Autodesk Inventor part; units mm, degrees
ref_plane "YZ Plane" through (0, 0, 0) normal (1, 0, 0) x (0, 1, 0)
ref_plane "XZ Plane" through (0, 0, 0) normal (0, 1, 0) x (-1, 0, 0)
ref_plane "XY Plane" through (0, 0, 0) normal (0, 0, 1) x (1, 0, 0)
sketch "main" plane through (0, 0, 0) normal (0, 0, 1) x (1, 0, 0)
  circle A0 centre (-11.9584, 56.4908) radius 2.1844
  circle A1 centre (13.4416, 56.4908) radius 2.1844
  circle A2 centre (13.4416, -57.8092) radius 2.1844
  circle A3 centre (-11.9584, -57.8092) radius 2.1844
  arc A4 (19.7916, 56.4908) -> (13.4416, 62.8408) centre (13.4416, 56.4908) ccw
  arc A5 (-11.9584, 62.8408) -> (-18.3084, 56.4908) centre (-11.9584, 56.4908) ccw
  arc A6 (-18.3084, -57.8092) -> (-11.9584, -64.1592) centre (-11.9584, -57.8092) ccw
  arc A7 (13.4416, -64.1592) -> (19.7916, -57.8092) centre (13.4416, -57.8092) ccw
  line L0 (13.4416, 62.8408) -> (-11.9584, 62.8408)
  line L1 (-18.3084, 56.4908) -> (-18.3084, -57.8092)
  line L2 (-11.9584, -64.1592) -> (13.4416, -64.1592)
  line L3 (19.7916, -57.8092) -> (19.7916, 56.4908)
  point P0 (0.7416, -0.6592)
  dimension "d0" = 12.7
  dimension "d1" = 12.7
  dimension "d2" = 12.7
  dimension "d3" = 12.7
sketch "Sketch1" plane through (0, 0, 0) normal (0, 1, 0) x (-1, 0, 0)
  circle A0 centre (-25.4, 0) radius 2.1844
  circle A1 centre (0, 0) radius 2.1844
  circle A2 centre (0, -114.3) radius 2.1844
  circle A3 centre (-25.4, -114.3) radius 2.1844
  arc A4 (6.35, 0) -> (0, 6.35) centre (0, 0) ccw
  arc A5 (-25.4, 6.35) -> (-31.75, 0) centre (-25.4, 0) ccw
  arc A6 (-31.75, -114.3) -> (-25.4, -120.65) centre (-25.4, -114.3) ccw
  arc A7 (0, -120.65) -> (6.35, -114.3) centre (0, -114.3) ccw
  line L0 (0, 6.35) -> (-25.4, 6.35)
  line L1 (-31.75, 0) -> (-31.75, -114.3)
  line L2 (-25.4, -120.65) -> (0, -120.65)
  line L3 (6.35, -114.3) -> (6.35, 0)
extrude "Extrusion1" add sketch "Sketch1" along normal blind 1.5875
properties part number "Brace Gusset" material "Acetal Resin, White"
Part model, mm, in its own coordinate system. Round coordinates to 2 decimals unless told otherwise and drop trailing zeros. Write each loop counter-clockwise with the first axis right and the second up, starting at its lowest first coordinate (ties: lowest second). Pieces come first, ordered by that corner, then holes. Notation, with made-up numbers: M -12.75,62 L -1.75,62 A26 cw -1.75,91 Z; hole C -27.75,56.25 d2. An arc over 180 degrees is marked long. Return JSON: item names as keys, results as strings. Group by question number.
(1) Two-plate mould, pull along X, no slides. Class faces 1 (the face through (13, 1.588, -56)), 2 (the face through (-4.44, 0.78, 4.54)), 3 (the face through (23.382, 0.783, 0.837)): +X half, -X half, draft (parallel to the pull), parting line (faces both ways), or undercut.
(2) Drill centre line: probe 1 along Z at (x, y) = (0, 0.6). Where is it in solid material? Low to high.
(3) Saw through at A-A on y = 0.8. Write the cut outline in (x, z).
(4) Pin check, flat tip, straight feed: pin 1 Ø7 at (x, z) = (25.4, -114.3) entering from +Y. Stop position of the tip, or through.
Returned:
{
 "1": {"face 1": "draft", "face 2": "-X half", "face 3": "undercut"},
 "2": {"probe 1": "-120.65 to -116.48, -112.12 to -2.18, 2.18 to 6.35"},
 "3": {"outline": "M -6.35,-114.3 A6.35 ccw 0,-120.65 L 25.4,-120.65 A6.35 ccw 31.75,-114.3 L 31.75,0 A6.35 ccw 25.4,6.35 L 0,6.35 A6.35 ccw -6.35,0 Z; hole C 0,-114.3 d4.37; hole C 0,0 d4.37; hole C 25.4,-114.3 d4.37; hole C 25.4,0 d4.37"},
 "4": {"pin 1": "y = 1.59"}
}
